Answer from the drawing. Dimensions are ordinates in mm from the lowest x, y and z of the part. A direction names the side the tool comes from. Give positions to 0.01 mm unless a question says otherwise; leave off trailing zeros. Order: outer loops, then holes, each group sorted by start corner. A loop starts at its lowest first (then second) coordinate and runs counter-clockwise, first axis right, second up.
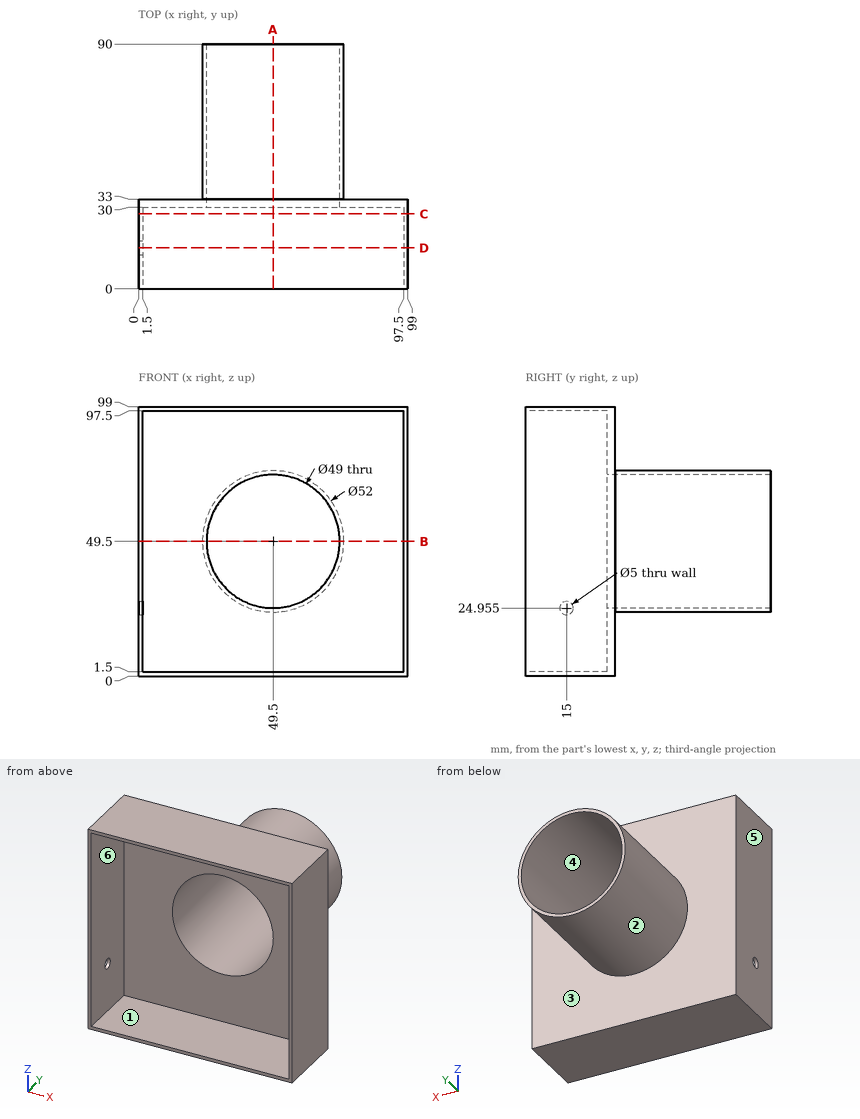
1. The part is cut by section C-C (y = 27.5). Write down the section's boundary in (x, z), then the cut area to 3 significant figures.
Findings below:
outline: (0, 0) - (99, 0) - (99, 99) - (0, 99) - close; hole (1.5, 1.5) - (97.5, 1.5) - (97.5, 97.5) - (1.5, 97.5) - close
area: 585 mm2
2. The part is cut by section B-B (z = 49.5). Write down the section's boundary in (x, y).
Findings below:
outline: (0, 0) - (1.5, 0) - (1.5, 30) - (25, 30) - (25, 90) - (23.5, 90) - (23.5, 33) - (0, 33) - close; (74, 30) - (97.5, 30) - (97.5, 0) - (99, 0) - (99, 33) - (75.5, 33) - (75.5, 90) - (74, 90) - close
3. Given P1, Ø1, axis at y = 61.5, z = 52, coming from the -X side; P2, Ø12, axis at y = 49, z = 58, coming from the +X side; P3, Ø10, axis at y = 57, z = 28, coming from the +X side, each flat-ended and moving along its own axis, determine where each tip first touches the part or whether it passes through.
Findings below:
P1: stops at x = 23.58
P2: stops at x = 75.38
P3: stops at x = 69.59
4. Straight lines are drawn through the part: probe 1 along Z at (x, y) = (49, 53); probe 2 along X at (y, z) = (7.5, 86). For each, find the intervals that lie inside material, in ascending order.
Findings below:
probe 1: z = 23.5 to 25.01, 73.99 to 75.5
probe 2: x = 0 to 1.5, 97.5 to 99
5. The part is cut by section A-A (x = 49.5). Write down the section's boundary in (y, z).
Findings below:
outline: (0, 0) - (33, 0) - (33, 23.5) - (90, 23.5) - (90, 25) - (30, 25) - (30, 1.5) - (0, 1.5) - close; (0, 97.5) - (30, 97.5) - (30, 74) - (90, 74) - (90, 75.5) - (33, 75.5) - (33, 99) - (0, 99) - close
6. Which of the six approach directions +Z, -Z, +X, -X, +Y, -Y give full straight-line access (tool end or side, diameter ignored) to the marked faces 5 and 6?
Findings below:
face 5: +Z, -Z, -X, +Y, -Y
face 6: -Y
7. The part is cut by section D-D (y = 15). Write down the section's boundary in (x, z) (3 decimals).
Findings below:
outline: (0, 0) - (99, 0) - (99, 99) - (0, 99) - (0, 27.455) - (1.5, 27.455) - (1.5, 97.5) - (97.5, 97.5) - (97.5, 1.5) - (1.5, 1.5) - (1.5, 22.455) - (0, 22.455) - close
8. The mould has two halves that part along X. Classify the marked faces 1, 2, 3 and 4: pulls with the +X half, pulls with the -X half, needs draft (parallel to the pull), parting line crosses it, or undercut.
Findings below:
face 1: undercut
face 2: parting line crosses it
face 3: needs draft
face 4: undercut
